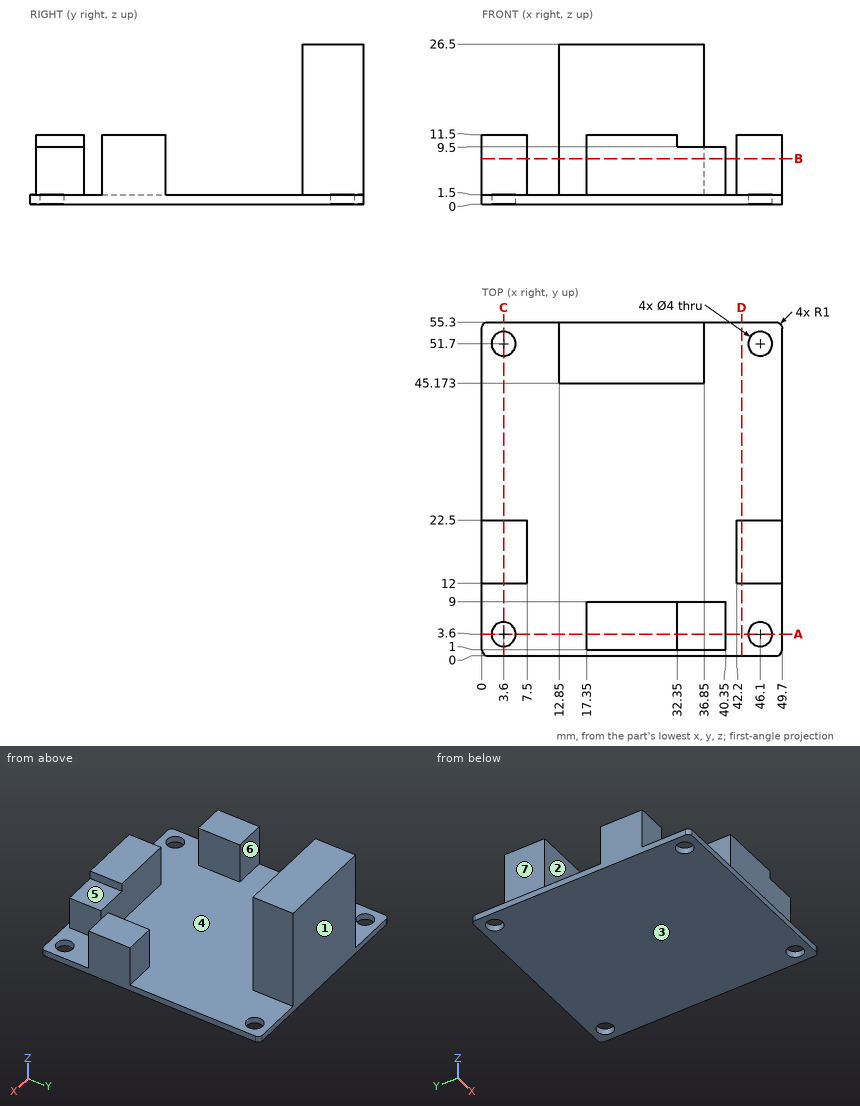
Design review of the part shown in the three views and the two pictorial views. Dimensions are in mm from the part's minimum x, y and z. A direction names the side the tool comes from. Round coordinates to 2 decimals unless told otherwise and drop trailing zeros. Order: outer loops, then holes, each group sorted by start corner. A loop starts at its lowest first (then second) coordinate and runs counter-clockwise, first axis right, second up.
(1) Take a section at B-B, the plane z = 7.5. State the section outline as (x, y) points.
Working result:
outline: (0, 12) - (7.5, 12) - (7.5, 22.5) - (0, 22.5) - close; (12.85, 45.17) - (36.85, 45.17) - (36.85, 55.3) - (12.85, 55.3) - close; (17.35, 1) - (40.35, 1) - (40.35, 9) - (17.35, 9) - close; (42.2, 12) - (49.7, 12) - (49.7, 22.5) - (42.2, 22.5) - close
(2) Wall thickness on L1, parallel to Y at x = 3.6, z = 1.25; L2, parallel to Y at x = 26.5, z = 6.25; L3, parallel to Z at x = 11, y = 39: over which ranges is each line inside the solid? List them lowest first.
Working result:
L1: y = 0 to 1.6, 5.6 to 49.7, 53.7 to 55.3
L2: y = 1 to 9, 45.17 to 55.3
L3: z = 0 to 1.5
(3) Take a section at D-D, the plane x = 43. State the section outline as (y, z) points.
Working result:
outline: (0, 0) - (55.3, 0) - (55.3, 1.5) - (22.5, 1.5) - (22.5, 11.5) - (12, 11.5) - (12, 1.5) - (0, 1.5) - close
(4) Tool access review of the marked faces 5, 6 and 7: name each direction out of +Z, -Z, +X, -X, +Y, -Y from which nothing blocks a thin tool from reaching the whole face with its end or side.
Working result:
face 5: +Z, +X, -Y
face 6: +Z, +X, -X, +Y
face 7: +Z, -X, +Y, -Y
(5) Mouldability with a two-part tool opening along Y and no side actions: class the marked faces 1, 2, 3 and 4 as released by +Y, released by -Y, zero draft, split by the parting line, or undercut.
Working result:
face 1: released by +Y
face 2: undercut
face 3: zero draft
face 4: undercut
(6) Take a section at A-A, the plane y = 3.6. State the section outline as (x, z) points.
Working result:
outline: (0, 0) - (1.6, 0) - (1.6, 1.5) - (0, 1.5) - close; (5.6, 0) - (44.1, 0) - (44.1, 1.5) - (40.35, 1.5) - (40.35, 9.5) - (32.35, 9.5) - (32.35, 11.5) - (17.35, 11.5) - (17.35, 1.5) - (5.6, 1.5) - close; (48.1, 0) - (49.7, 0) - (49.7, 1.5) - (48.1, 1.5) - close
(7) For P1, Ø3, axis at y = 50, z = 11.5, coming from the +X side; P2, Ø4, axis at x = 36.5, y = 5.5, coming from the +Z side; P3, Ø2.5, axis at y = 3.5, z = 8, coming from the -X side; P4, Ø10, axis at y = 37, z = 9, coming from the +X side, all flat-tipped, find the tip position at first contact; note any pin that passes through.
Working result:
P1: stops at x = 36.85
P2: stops at z = 9.5
P3: stops at x = 17.35
P4: passes through
(8) Take a section at C-C, the plane x = 3.6. State the section outline as (y, z) points, plus the area to 3 significant figures.
Working result:
outline: (0, 0) - (1.6, 0) - (1.6, 1.5) - (0, 1.5) - close; (5.6, 0) - (49.7, 0) - (49.7, 1.5) - (22.5, 1.5) - (22.5, 11.5) - (12, 11.5) - (12, 1.5) - (5.6, 1.5) - close; (53.7, 0) - (55.3, 0) - (55.3, 1.5) - (53.7, 1.5) - close
area: 176 mm2
